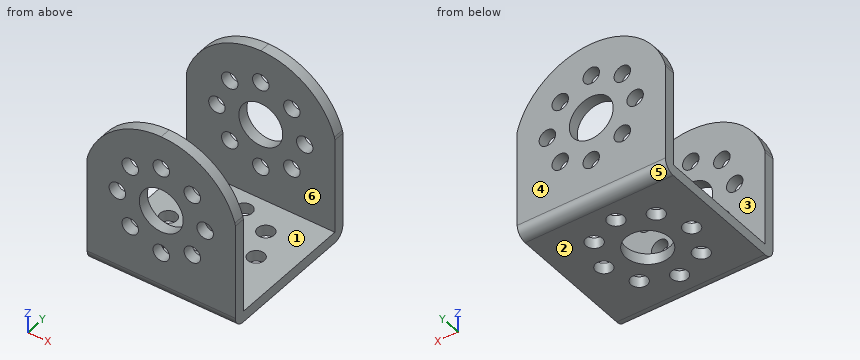
from build123d import *

# Parameters (mm, degrees)
F1_DEPTH = 27
F2_R     = 1.5
F2_R_2   = 4
F3_DEPTH = 27.001
F5_DEPTH = 27.001
F6_R     = 2
F7_R     = 4
F7_R_2   = 1.5
F8_DEPTH = 25


with BuildPart() as f1:
    # F0 (on Right) → F1 (new body)
    with BuildSketch(Plane.YZ):
        Polygon((0, 30), (0, 0), (27, 0), (27, 30), (25, 30), (25, 2), (2, 2), (2, 30), align=None)
    extrude(amount=F1_DEPTH)

    # F2 (on face) → F3 (cut, through all)
    with BuildSketch(Plane(origin=(0, 27, 0), x_dir=(-1, 0, 0), z_dir=(0, 1, 0))):
        with Locations((-13.5, 24)):
            Circle(F2_R)
        with Locations((-7.8431457505, 21.6568542495)):
            Circle(F2_R)
        with Locations((-5.5, 16)):
            Circle(F2_R)
        with Locations((-7.8431457505, 10.3431457505)):
            Circle(F2_R)
        with Locations((-13.5, 8)):
            Circle(F2_R)
        with Locations((-19.1568542495, 10.3431457505)):
            Circle(F2_R)
        with Locations((-21.5, 16)):
            Circle(F2_R)
        with Locations((-13.5, 16)):
            Circle(F2_R_2)
        with Locations((-19.1568542495, 21.6568542495)):
            Circle(F2_R)
    extrude(amount=-F3_DEPTH, mode=Mode.SUBTRACT)

    # F4 (on face) → F5 (cut, through all)
    with BuildSketch(Plane(origin=(0, 27, 0), x_dir=(-1, 0, 0), z_dir=(0, 1, 0))):
        with BuildLine():
            ThreePointArc((-27, 19.7080992435), (-21.9878327796, 27.1335840907), (-13.5, 30))
            Line((-13.5, 30), (-27, 30))
            Line((-27, 30), (-27, 19.7080992435))
        make_face()
        with BuildLine():
            ThreePointArc((-13.5, 30), (-5.0121672204, 27.1335840907), (0, 19.7080992435))
            Line((0, 19.7080992435), (0, 30))
            Line((0, 30), (-13.5, 30))
        make_face()
    extrude(amount=-F5_DEPTH, mode=Mode.SUBTRACT)

    # F6
    f6_edges = [f1.edges().sort_by_distance(p)[0] for p in [
        (27, 1, 19.708099),
        (0, 1, 19.708099),
        (0, 26, 19.708099),
        (27, 26, 19.708099),
        (13.5, 27, 0),
        (13.5, 0, 0),
    ]]
    fillet(f6_edges, radius=F6_R)

    # F7 (on face) → F8 (cut)
    with BuildSketch(Plane(origin=(0, 0, 0), x_dir=(1, 0, 0), z_dir=(0, 0, -1))):
        with Locations((13, -13.5)):
            Circle(F7_R)
        with Locations((21, -13.5)):
            Circle(F7_R_2)
        with Locations((18.6568542495, -19.1568542495)):
            Circle(F7_R_2)
        with Locations((13, -21.5)):
            Circle(F7_R_2)
        with Locations((7.3431457505, -19.1568542495)):
            Circle(F7_R_2)
        with Locations((5, -13.5)):
            Circle(F7_R_2)
        with Locations((7.3431457505, -7.8431457505)):
            Circle(F7_R_2)
        with Locations((13, -5.5)):
            Circle(F7_R_2)
        with Locations((18.6568542495, -7.8431457505)):
            Circle(F7_R_2)
    extrude(amount=-F8_DEPTH, mode=Mode.SUBTRACT)


solid = f1.part
Can you work these out from the model? Positions are in its coordinate system, mm. Face numbers are marked on the shaded views. A direction names the side the tool comes from. Round coordinates to 2 decimals unless told otherwise and drop trailing zeros. Write each loop counter-clockwise with the first axis right and the second up, starting at its lowest first coordinate (ties: lowest second). Pieces come first, ordered by that corner, then holes. Notation, with made-up numbers: (69, -21.5) - (88, -21.5) arc R25 cw to (88, 7.5) - close; hole circle Ø4 at (53, -7.5). An arc over 180 degrees is marked (long way). Write each question's results on one line, items separated by ' | '. Start each with the question number.
1) For pin 1 Ø4 at (x, y) = (5, 13.5) entering from +Z, with a flat end and sliding along its axis, tell me the tip position at first contact or that it passes through.
2) Which directions (+Z, -Z, +X, -X, +Y, -Y) give clear straight access to the entire face, cutting with the end or side of a thin tool? Please do the marked faces 5 and 6.
3) Please list where these lines run through material, in increasing order: line 1 (Y direction, x = 7.25, z = 25.5); line 2 (X direction, y = 5.5, z = 1.1); line 3 (Z direction, x = 12.5, y = 7).
4) Suppose I cut it at D-D (x = 18.25). Give the number of separate pieces and of enclosed holes in the cut face, and give its area (3 significant figures).
5) Suppose I cut it at A-A (z = 8). List the corners of the cut face in (x, y) for me.
6) We'd pull the mould along Y, two halves only. Please class the marked faces 1, 2, 3 and 4: released by +Y, released by -Y, zero draft, split by the parting line, or undercut.
7) Suppose I cut it at C-C (x = 21.5). List the corners of the cut face in (y, z) for me.
8) Suppose I cut it at B-B (y = 21.5). List the corners of the cut face in (x, z) for me, and give its area (3 significant figures).
Here are the results:
1) pin 1: stops at z = 2
2) face 5: -Z, +X, -X, +Y | face 6: +Z, +X, -X
3) line 1: y = 0 to 2, 25 to 27 | line 2: x = 0 to 11.5, 14.5 to 27 | line 3: z = 0 to 2
4) separate pieces: 7 | enclosed holes: 0 | area: 130 mm2
5) outline: (0, 0) - (12, 0) - (12, 2) - (0, 2) - close; (0, 25) - (12, 25) - (12, 27) - (0, 27) - close; (15, 0) - (27, 0) - (27, 2) - (15, 2) - close; (15, 25) - (27, 25) - (27, 27) - (15, 27) - close
6) face 1: undercut | face 2: zero draft | face 3: undercut | face 4: released by +Y
7) outline: (0, 2) arc R2 ccw to (2, 0) - (12.09, 0) - (12.09, 2) - (2, 2) - (2, 14.5) - (0, 14.5) - close; (0, 17.5) - (2, 17.5) - (2, 27.49) - (0, 27.49) - close; (14.91, 0) - (25, 0) arc R2 ccw to (27, 2) - (27, 14.5) - (25, 14.5) - (25, 2) - (14.91, 2) - close; (25, 17.5) - (27, 17.5) - (27, 27.49) - (25, 27.49) - close
8) outline: (0, 0) - (11.5, 0) - (11.5, 2) - (0, 2) - close; (14.5, 0) - (27, 0) - (27, 2) - (14.5, 2) - close | area: 48.0 mm2
